```python
from build123d import *

# Parameters (mm, degrees)
SKETCH1_R              = 3
BOSS_EXTRUDE2_DEPTH    = 29
BOSS_EXTRUDE2_2_DEPTH  = 29
BOSS_EXTRUDE2_3_DEPTH  = 29
BOSS_EXTRUDE2_4_DEPTH  = 29
BOSS_EXTRUDE2_5_DEPTH  = 29
BOSS_EXTRUDE2_6_DEPTH  = 29
BOSS_EXTRUDE2_7_DEPTH  = 29
BOSS_EXTRUDE2_8_DEPTH  = 29
BOSS_EXTRUDE2_9_DEPTH  = 29
BOSS_EXTRUDE2_10_DEPTH = 29
BOSS_EXTRUDE2_11_DEPTH = 29
BOSS_EXTRUDE2_12_DEPTH = 29
BOSS_EXTRUDE2_13_DEPTH = 29
BOSS_EXTRUDE2_14_DEPTH = 29
BOSS_EXTRUDE2_15_DEPTH = 29
BOSS_EXTRUDE2_16_DEPTH = 29
SKETCH2_R              = 47.85
SKETCH2_R_2            = 46.5
BOSS_EXTRUDE4_DEPTH    = 29
SKETCH3_R              = 46.5
CUT_EXTRUDE1_DEPTH     = 3
SKETCH4_R              = 46.5
CUT_EXTRUDE2_DEPTH     = 3
SKETCH5_R              = 48.35
SKETCH5_R_2            = 47.85
BOSS_EXTRUDE6_DEPTH    = 29


with BuildPart() as part:
    # Sketch1 → Boss-Extrude2 (new body)
    with BuildSketch(Plane.XY):
        with Locations((-41.435997033, 17.163351942)):
            Circle(SKETCH1_R)
    extrude(amount=BOSS_EXTRUDE2_DEPTH)


with BuildPart() as body_2:
    # Sketch1 → Boss-Extrude2 2 (new body)
    with BuildSketch(Plane.XY):
        with Locations((-31.713739136, 31.713739136)):
            Circle(SKETCH1_R)
    extrude(amount=BOSS_EXTRUDE2_2_DEPTH)


with BuildPart() as body_3:
    # Sketch1 → Boss-Extrude2 3 (new body)
    with BuildSketch(Plane.XY):
        with Locations((-17.163351942, 41.435997033)):
            Circle(SKETCH1_R)
    extrude(amount=BOSS_EXTRUDE2_3_DEPTH)


with BuildPart() as body_4:
    # Sketch1 → Boss-Extrude2 4 (new body)
    with BuildSketch(Plane.XY):
        with Locations((0, 44.85)):
            Circle(SKETCH1_R)
    extrude(amount=BOSS_EXTRUDE2_4_DEPTH)


with BuildPart() as body_5:
    # Sketch1 → Boss-Extrude2 5 (new body)
    with BuildSketch(Plane.XY):
        with Locations((17.163351942, 41.435997033)):
            Circle(SKETCH1_R)
    extrude(amount=BOSS_EXTRUDE2_5_DEPTH)


with BuildPart() as body_6:
    # Sketch1 → Boss-Extrude2 6 (new body)
    with BuildSketch(Plane.XY):
        with Locations((31.713739136, 31.713739136)):
            Circle(SKETCH1_R)
    extrude(amount=BOSS_EXTRUDE2_6_DEPTH)


with BuildPart() as body_7:
    # Sketch1 → Boss-Extrude2 7 (new body)
    with BuildSketch(Plane.XY):
        with Locations((41.435997033, 17.163351942)):
            Circle(SKETCH1_R)
    extrude(amount=BOSS_EXTRUDE2_7_DEPTH)


with BuildPart() as body_8:
    # Sketch1 → Boss-Extrude2 8 (new body)
    with BuildSketch(Plane.XY):
        with Locations((44.85, 0)):
            Circle(SKETCH1_R)
    extrude(amount=BOSS_EXTRUDE2_8_DEPTH)


with BuildPart() as body_9:
    # Sketch1 → Boss-Extrude2 9 (new body)
    with BuildSketch(Plane.XY):
        with Locations((41.435997033, -17.163351942)):
            Circle(SKETCH1_R)
    extrude(amount=BOSS_EXTRUDE2_9_DEPTH)


with BuildPart() as body_10:
    # Sketch1 → Boss-Extrude2 10 (new body)
    with BuildSketch(Plane.XY):
        with Locations((17.163351942, -41.435997033)):
            Circle(SKETCH1_R)
    extrude(amount=BOSS_EXTRUDE2_10_DEPTH)


with BuildPart() as body_11:
    # Sketch1 → Boss-Extrude2 11 (new body)
    with BuildSketch(Plane.XY):
        with Locations((0, -44.85)):
            Circle(SKETCH1_R)
    extrude(amount=BOSS_EXTRUDE2_11_DEPTH)


with BuildPart() as body_12:
    # Sketch1 → Boss-Extrude2 12 (new body)
    with BuildSketch(Plane.XY):
        with Locations((-17.163351942, -41.435997033)):
            Circle(SKETCH1_R)
    extrude(amount=BOSS_EXTRUDE2_12_DEPTH)


with BuildPart() as body_13:
    # Sketch1 → Boss-Extrude2 13 (new body)
    with BuildSketch(Plane.XY):
        with Locations((-41.435997033, -17.163351942)):
            Circle(SKETCH1_R)
    extrude(amount=BOSS_EXTRUDE2_13_DEPTH)


with BuildPart() as body_14:
    # Sketch1 → Boss-Extrude2 14 (new body)
    with BuildSketch(Plane.XY):
        with Locations((-31.713739136, -31.713739136)):
            Circle(SKETCH1_R)
    extrude(amount=BOSS_EXTRUDE2_14_DEPTH)


with BuildPart() as body_15:
    # Sketch1 → Boss-Extrude2 15 (new body)
    with BuildSketch(Plane.XY):
        with Locations((-44.85, 0)):
            Circle(SKETCH1_R)
    extrude(amount=BOSS_EXTRUDE2_15_DEPTH)


with BuildPart() as body_16:
    # Sketch1 → Boss-Extrude2 16 (new body)
    with BuildSketch(Plane.XY):
        with Locations((31.713739136, -31.713739136)):
            Circle(SKETCH1_R)
    extrude(amount=BOSS_EXTRUDE2_16_DEPTH)


with BuildPart() as body_17:
    # Sketch2 → Boss-Extrude4 (new body)
    with BuildSketch(Plane(origin=(0, 0, 0), x_dir=(-1, 0, 0), z_dir=(0, 0, -1))):
        Circle(SKETCH2_R)
        Circle(SKETCH2_R_2, mode=Mode.SUBTRACT)
    extrude(amount=-BOSS_EXTRUDE4_DEPTH)


with BuildPart() as cut_extrude1_tool:
    # Sketch3 → Cut-Extrude1 (new body)
    with BuildSketch(Plane(origin=(0, 0, 0), x_dir=(-1, 0, 0), z_dir=(0, 0, -1))):
        Circle(SKETCH3_R)
    extrude(amount=-CUT_EXTRUDE1_DEPTH)


with BuildPart() as part_1:
    add(part.part)

    # Cut-Extrude1: cut by cut_extrude1_tool
    add(cut_extrude1_tool.part, mode=Mode.SUBTRACT)


with BuildPart() as body_2_1:
    add(body_2.part)

    # Cut-Extrude1: cut by cut_extrude1_tool
    add(cut_extrude1_tool.part, mode=Mode.SUBTRACT)


with BuildPart() as body_3_1:
    add(body_3.part)

    # Cut-Extrude1: cut by cut_extrude1_tool
    add(cut_extrude1_tool.part, mode=Mode.SUBTRACT)


with BuildPart() as body_4_1:
    add(body_4.part)

    # Cut-Extrude1: cut by cut_extrude1_tool
    add(cut_extrude1_tool.part, mode=Mode.SUBTRACT)


with BuildPart() as body_5_1:
    add(body_5.part)

    # Cut-Extrude1: cut by cut_extrude1_tool
    add(cut_extrude1_tool.part, mode=Mode.SUBTRACT)


with BuildPart() as body_6_1:
    add(body_6.part)

    # Cut-Extrude1: cut by cut_extrude1_tool
    add(cut_extrude1_tool.part, mode=Mode.SUBTRACT)


with BuildPart() as body_7_1:
    add(body_7.part)

    # Cut-Extrude1: cut by cut_extrude1_tool
    add(cut_extrude1_tool.part, mode=Mode.SUBTRACT)


with BuildPart() as body_8_1:
    add(body_8.part)

    # Cut-Extrude1: cut by cut_extrude1_tool
    add(cut_extrude1_tool.part, mode=Mode.SUBTRACT)


with BuildPart() as body_9_1:
    add(body_9.part)

    # Cut-Extrude1: cut by cut_extrude1_tool
    add(cut_extrude1_tool.part, mode=Mode.SUBTRACT)


with BuildPart() as body_10_1:
    add(body_10.part)

    # Cut-Extrude1: cut by cut_extrude1_tool
    add(cut_extrude1_tool.part, mode=Mode.SUBTRACT)


with BuildPart() as body_11_1:
    add(body_11.part)

    # Cut-Extrude1: cut by cut_extrude1_tool
    add(cut_extrude1_tool.part, mode=Mode.SUBTRACT)


with BuildPart() as body_12_1:
    add(body_12.part)

    # Cut-Extrude1: cut by cut_extrude1_tool
    add(cut_extrude1_tool.part, mode=Mode.SUBTRACT)


with BuildPart() as body_13_1:
    add(body_13.part)

    # Cut-Extrude1: cut by cut_extrude1_tool
    add(cut_extrude1_tool.part, mode=Mode.SUBTRACT)


with BuildPart() as body_14_1:
    add(body_14.part)

    # Cut-Extrude1: cut by cut_extrude1_tool
    add(cut_extrude1_tool.part, mode=Mode.SUBTRACT)


with BuildPart() as body_15_1:
    add(body_15.part)

    # Cut-Extrude1: cut by cut_extrude1_tool
    add(cut_extrude1_tool.part, mode=Mode.SUBTRACT)


with BuildPart() as body_16_1:
    add(body_16.part)

    # Cut-Extrude1: cut by cut_extrude1_tool
    add(cut_extrude1_tool.part, mode=Mode.SUBTRACT)


with BuildPart() as cut_extrude2_tool:
    # Sketch4 → Cut-Extrude2 (new body)
    with BuildSketch(Plane.XY.offset(29)):
        Circle(SKETCH4_R)
    extrude(amount=-CUT_EXTRUDE2_DEPTH)


with BuildPart() as part_2:
    add(part_1.part)

    # Cut-Extrude2: cut by cut_extrude2_tool
    add(cut_extrude2_tool.part, mode=Mode.SUBTRACT)



with BuildPart() as body_2_2:
    add(body_2_1.part)

    # Cut-Extrude2: cut by cut_extrude2_tool
    add(cut_extrude2_tool.part, mode=Mode.SUBTRACT)


with BuildPart() as body_3_2:
    add(body_3_1.part)

    # Cut-Extrude2: cut by cut_extrude2_tool
    add(cut_extrude2_tool.part, mode=Mode.SUBTRACT)


with BuildPart() as body_4_2:
    add(body_4_1.part)

    # Cut-Extrude2: cut by cut_extrude2_tool
    add(cut_extrude2_tool.part, mode=Mode.SUBTRACT)


with BuildPart() as body_5_2:
    add(body_5_1.part)

    # Cut-Extrude2: cut by cut_extrude2_tool
    add(cut_extrude2_tool.part, mode=Mode.SUBTRACT)


with BuildPart() as body_6_2:
    add(body_6_1.part)

    # Cut-Extrude2: cut by cut_extrude2_tool
    add(cut_extrude2_tool.part, mode=Mode.SUBTRACT)


with BuildPart() as body_7_2:
    add(body_7_1.part)

    # Cut-Extrude2: cut by cut_extrude2_tool
    add(cut_extrude2_tool.part, mode=Mode.SUBTRACT)


with BuildPart() as body_8_2:
    add(body_8_1.part)

    # Cut-Extrude2: cut by cut_extrude2_tool
    add(cut_extrude2_tool.part, mode=Mode.SUBTRACT)


with BuildPart() as body_9_2:
    add(body_9_1.part)

    # Cut-Extrude2: cut by cut_extrude2_tool
    add(cut_extrude2_tool.part, mode=Mode.SUBTRACT)


with BuildPart() as body_10_2:
    add(body_10_1.part)

    # Cut-Extrude2: cut by cut_extrude2_tool
    add(cut_extrude2_tool.part, mode=Mode.SUBTRACT)


with BuildPart() as body_11_2:
    add(body_11_1.part)

    # Cut-Extrude2: cut by cut_extrude2_tool
    add(cut_extrude2_tool.part, mode=Mode.SUBTRACT)


with BuildPart() as body_12_2:
    add(body_12_1.part)

    # Cut-Extrude2: cut by cut_extrude2_tool
    add(cut_extrude2_tool.part, mode=Mode.SUBTRACT)


with BuildPart() as body_13_2:
    add(body_13_1.part)

    # Cut-Extrude2: cut by cut_extrude2_tool
    add(cut_extrude2_tool.part, mode=Mode.SUBTRACT)


with BuildPart() as body_14_2:
    add(body_14_1.part)

    # Cut-Extrude2: cut by cut_extrude2_tool
    add(cut_extrude2_tool.part, mode=Mode.SUBTRACT)


with BuildPart() as body_15_2:
    add(body_15_1.part)

    # Cut-Extrude2: cut by cut_extrude2_tool
    add(cut_extrude2_tool.part, mode=Mode.SUBTRACT)


with BuildPart() as body_16_2:
    add(body_16_1.part)

    # Cut-Extrude2: cut by cut_extrude2_tool
    add(cut_extrude2_tool.part, mode=Mode.SUBTRACT)


with BuildPart() as part_3:
    add(part_2.part)

    add(body_2_2.part)  # Boss-Extrude6 merges body 2

    add(body_3_2.part)  # Boss-Extrude6 merges body 3

    add(body_4_2.part)  # Boss-Extrude6 merges body 4

    add(body_5_2.part)  # Boss-Extrude6 merges body 5

    add(body_6_2.part)  # Boss-Extrude6 merges body 6

    add(body_7_2.part)  # Boss-Extrude6 merges body 7

    add(body_8_2.part)  # Boss-Extrude6 merges body 8

    add(body_9_2.part)  # Boss-Extrude6 merges body 9

    add(body_10_2.part)  # Boss-Extrude6 merges body 10

    add(body_11_2.part)  # Boss-Extrude6 merges body 11

    add(body_12_2.part)  # Boss-Extrude6 merges body 12

    add(body_13_2.part)  # Boss-Extrude6 merges body 13

    add(body_14_2.part)  # Boss-Extrude6 merges body 14

    add(body_15_2.part)  # Boss-Extrude6 merges body 15

    add(body_16_2.part)  # Boss-Extrude6 merges body 16

    add(body_17.part)  # Boss-Extrude6 merges body 17
    # Sketch5 → Boss-Extrude6 (add)
    with BuildSketch(Plane(origin=(0, 0, 0), x_dir=(-1, 0, 0), z_dir=(0, 0, -1))):
        Circle(SKETCH5_R)
        Circle(SKETCH5_R_2, mode=Mode.SUBTRACT)
    extrude(amount=-BOSS_EXTRUDE6_DEPTH)


solid = part_3.part
```
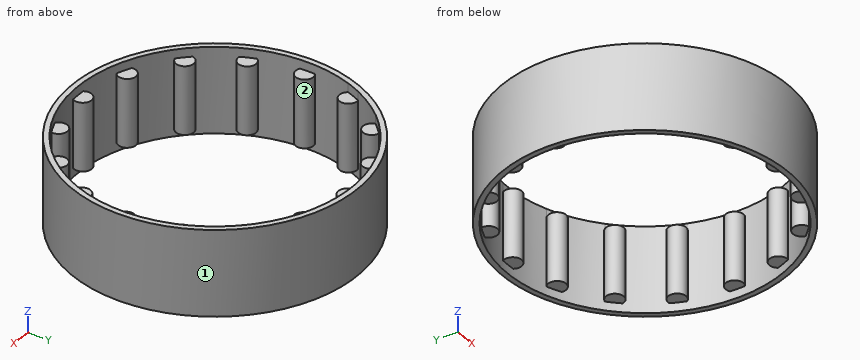
Work out the finished part from the listing and answer in its coordinate system (mm). Face numbers are marked on the shaded views. Give positions to 0.01 mm unless a question says otherwise; leave off trailing zeros. Loops run counter-clockwise (first coordinate to the right, second up) from the corner with the lowest first, then second, coordinate; pieces in that order, holes last. Notation, with made-up numbers: M 0,52 L 41,52 A25 cw 41,80 Z; hole C 73.25,18 d3. An arc over 180 degrees is marked long. One line per item, written item: value. Start each with the question number.
1. Find section A-A (x = 0). Give the vertices of the cut face in (y, z), and give its area (3 significant figures).
2. Find the intervals of material crossed by probe 1 along X at (y, z) = (0.5, 24); probe 2 along Y at (x, z) = (40.5, 4); probe 3 along Y at (x, z) = (0, 8), in increasing order.
3. Find section B-B (y = -26). Give the vertices of the cut face in (x, z), and give its area (3 significant figures).
4. Find section D-D (x = -40). Give the vertices of the cut face in (y, z), and give its area (3 significant figures).
5. Determine the mould class of the marked faces 1 and 2 for opening direction X: released by +X, released by -X, zero draft, split by the parting line, or undercut.
6. Each of these flat-tipped pins is pushed along its axis until it touches: P1, Ø1.5, axis at x = -21, z = 3.5, coming from the +Y side; P2, Ø6, axis at x = -15.5, y = -40, coming from the -Z side; P3, Ø4.5, axis at x = 41, y = -16.5, coming from the +Z side; P4, Ø1.5, axis at x = -31.5, y = 26, coming from the -Z side. Where does it stop, or does it pass through?
Reported:
1. outline: M -48.35,0 L -46.5,0 L -46.5,3 L -41.85,3 L -41.85,26 L -46.5,26 L -46.5,29 L -48.35,29 Z; M 41.85,3 L 46.5,3 L 46.5,0 L 48.35,0 L 48.35,29 L 46.5,29 L 46.5,26 L 41.85,26 Z
1. area: 321 mm²
2. probe 1: x = -48.35 to -41.89, 41.89 to 48.35
2. probe 2: y = -26.41 to -22.85, -20.01 to -14.31, 14.31 to 20.01, 22.85 to 26.41
2. probe 3: y = -48.35 to -41.85, 41.85 to 48.35
3. outline: M -40.76,0 L -38.55,0 L -38.55,29 L -40.76,29 Z; M 38.55,0 L 40.76,0 L 40.76,29 L 38.55,29 Z
3. area: 128 mm²
4. outline: M -27.16,0 L -23.71,0 L -23.71,29 L -27.16,29 Z; M -19.8,3 L -14.53,3 L -14.53,26 L -19.8,26 Z; M 14.53,3 L 19.8,3 L 19.8,26 L 14.53,26 Z; M 23.71,0 L 27.16,0 L 27.16,29 L 23.71,29 Z
4. area: 442 mm²
5. face 1: split by the parting line
5. face 2: undercut
6. P1: stops at y = 43.91
6. P2: stops at z = 3
6. P3: stops at z = 26
6. P4: passes through
